Autodesk Inventor part; units mm, degrees
ref_plane "YZ Plane" through (0, 0, 0) normal (1, 0, 0) x (0, 1, 0)
ref_plane "XZ Plane" through (0, 0, 0) normal (0, 1, 0) x (-1, 0, 0)
ref_plane "XY Plane" through (0, 0, 0) normal (0, 0, 1) x (1, 0, 0)
sketch "Sketch1" plane through (0, 0, 0) normal (0, 1, 0) x (-1, 0, 0)
  line L0 (500, 500) -> (-500, 500)
  line L1 (-500, 500) -> (-500, -500)
  line L2 (-500, -500) -> (500, -500)
  line L3 (500, -500) -> (500, 500)
  point P0 (0, 0)
  point P1 (0, 500)
  point P2 (500, 0)
  dimension "d1" = 1000
  dimension "d2" = 1000
extrude "Extrusion1" add sketch "Sketch1" along normal blind 10
sketch "Sketch2" plane through (0, 10, 0) normal (0, 1, 0) x (1, 0, 0)
  line L0 (-480, -480) -> (480, -480)
  line L1 (480, -480) -> (480, 480)
  line L2 (480, 480) -> (-480, 480)
  line L3 (-480, 480) -> (-480, -480)
  line L4 (-500, 500) -> (-500, -500)
  line L5 (-500, -500) -> (500, -500)
  line L6 (500, -500) -> (500, 500)
  line L7 (500, 500) -> (-500, 500)
  point P0 (0, 0)
  dimension "d5" = 20
  dimension "d6" = 20
  dimension "d8" = 20
  dimension "d9" = 20
extrude "Extrusion2" add sketch "Sketch2" along normal blind 20
fillet "Fillet1" radius 100 4 edges at (-480, 20, 480) (-480, 20, -480) (480, 20, -480) (480, 20, 480)
fillet "Fillet2" radius 120 4 edges at (-500, 15, 500) (-500, 15, -500) (500, 15, -500) (500, 15, 500)
equation "\"d6\" = d5"
equation "\"d8\" = d5"
equation "\"d9\" = d5"
properties part number "ground"
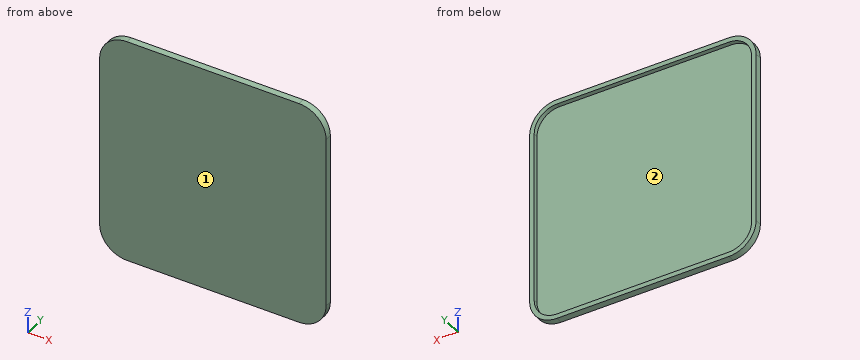
Model file for the job. Use its own axes, mm. Face numbers are marked on the shaded views. Round coordinates to 2 decimals unless told otherwise and drop trailing zeros. Loops run counter-clockwise (first coordinate to the right, second up) from the corner with the lowest first, then second, coordinate; pieces in that order, holes last.
1. Band-saw the part on A-A, the plane y = 20. List the corners of the cut face in (x, z), and give its area (3 significant figures).
Check values:
outline: (-500, -380) arc R120 ccw to (-380, -500) - (380, -500) arc R120 ccw to (500, -380) - (500, 380) arc R120 ccw to (380, 500) - (-380, 500) arc R120 ccw to (-500, 380) - close; hole (-480, -380) arc R100 ccw to (-380, -480) - (380, -480) arc R100 ccw to (480, -380) - (480, 380) arc R100 ccw to (380, 480) - (-380, 480) arc R100 ccw to (-480, 380) - close
area: 74,600 mm2
2. Drop a flat-ended pin along its axis: P1, Ø10, axis at x = -258.5, z = -100.5, coming from the +Y side. Give the stop position or say it passes through.
Check values:
P1: stops at y = 10
3. Band-saw the part on C-C, the plane z = 185. List the corners of the cut face in (x, y).
Check values:
outline: (-500, 0) - (500, 0) - (500, 30) - (480, 30) - (480, 10) - (-480, 10) - (-480, 30) - (-500, 30) - close
4. Band-saw the part on B-B, the plane x = -345. List the corners of the cut face in (y, z), and give its area (3 significant figures).
Check values:
outline: (0, -500) - (30, -500) - (30, -480) - (10, -480) - (10, 480) - (30, 480) - (30, 500) - (0, 500) - close
area: 10,800 mm2
5. Mould opens along Z. For the marked faces 1 and 2 say: +Z half, -Z half, draft (parallel to the pull), parting line (faces both ways), or undercut.
Check values:
face 1: draft
face 2: undercut
6. Wall check: probe 1 along X at (y, z) = (26, 284); probe 2 along Y at (x, z) = (-85, 268.5). Give the ranges that are in metal, low to high.
Check values:
probe 1: x = -500 to -480, 480 to 500
probe 2: y = 0 to 10
